```python
from build123d import *

# Parameters (mm, degrees)
BOSS_EXTRUDE1_DEPTH = 1.5875
SKETCH3_R           = 1.5
CUT_EXTRUDE1_DEPTH  = 1.5875
SKETCH4_W           = 8.5
SKETCH4_H           = 40
CUT_EXTRUDE2_DEPTH  = 52.910426175
CUT_EXTRUDE3_DEPTH  = 52.910426175


with BuildPart() as part:
    # Sketch2 → Boss-Extrude1 (new body)
    with BuildSketch(Plane.XY):
        with BuildLine():
            Line((41.075, 26.06487963), (34.753871084, 26.06487963))
            Line((34.753871084, 26.06487963), (34.753871084, 27.4075156))
            ThreePointArc((34.753871084, 27.4075156), (34.460977865, 28.114622381), (33.753871084, 28.4075156))
            Line((33.753871084, 28.4075156), (-33.743187521, 28.4075156))
            ThreePointArc((-33.743187521, 28.4075156), (-34.450294302, 28.114622381), (-34.743187521, 27.4075156))
            Line((-34.743187521, 27.4075156), (-34.743187521, 26.06487963))
            Line((-34.743187521, 26.06487963), (-41.075, 26.06487963))
            Line((-41.075, 26.06487963), (-41.075, 14.733067151))
            Line((-41.075, 14.733067151), (-42.4124996, 14.733067151))
            ThreePointArc((-42.4124996, 14.733067151), (-43.119606381, 14.440173932), (-43.4124996, 13.733067151))
            Line((-43.4124996, 13.733067151), (-43.4124996, -13.743187521))
            ThreePointArc((-43.4124996, -13.743187521), (-43.119606381, -14.450294302), (-42.4124996, -14.743187521))
            Line((-42.4124996, -14.743187521), (-41.075, -14.743187521))
            Line((-41.075, -14.743187521), (-41.075, -26.08512037))
            Line((-41.075, -26.08512037), (-29.75263109, -26.08512037))
            Line((-29.75263109, -26.08512037), (-29.75263109, -27.41690205))
            ThreePointArc((-29.75263109, -27.41690205), (-29.459737872, -28.124008831), (-28.75263109, -28.41690205))
            Line((-28.75263109, -28.41690205), (28.813455755, -28.41690205))
            ThreePointArc((28.813455755, -28.41690205), (29.520562536, -28.124008831), (29.813455755, -27.41690205))
            Line((29.813455755, -27.41690205), (29.813455755, -26.08512037))
            Line((29.813455755, -26.08512037), (41.075, -26.08512037))
            Line((41.075, -26.08512037), (41.075, -19.823575131))
            Line((41.075, -19.823575131), (42.412577294, -19.823575131))
            ThreePointArc((42.412577294, -19.823575131), (43.119684076, -19.530681912), (43.412577294, -18.823575131))
            Line((43.412577294, -18.823575131), (43.412577294, 18.721630511))
            ThreePointArc((43.412577294, 18.721630511), (43.119684076, 19.428737292), (42.412577294, 19.721630511))
            Line((42.412577294, 19.721630511), (41.075, 19.721630511))
            Line((41.075, 19.721630511), (41.075, 26.06487963))
        make_face()
    extrude(amount=BOSS_EXTRUDE1_DEPTH)

    # Sketch3 → Cut-Extrude1 (cut)
    with BuildSketch(Plane(origin=(0, 0, 0), x_dir=(-1, 0, 0), z_dir=(0, 0, -1))):
        with Locations((40.825, 25.825)):
            Circle(SKETCH3_R)
        with Locations((-40.825, 25.825)):
            Circle(SKETCH3_R)
        with Locations((-40.825, -25.825)):
            Circle(SKETCH3_R)
        with Locations((40.825, -25.825)):
            Circle(SKETCH3_R)
    extrude(amount=-CUT_EXTRUDE1_DEPTH, mode=Mode.SUBTRACT)

    # Sketch4 → Cut-Extrude2 (cut, through all)
    with BuildSketch(Plane(origin=(0, 0, 0), x_dir=(-1, 0, 0), z_dir=(0, 0, -1))):
        Polygon((-28.41, -20.51), (-28.41, 20.96), (34.89, 20.96), (34.89, -20.51), (34.89, -22.36), (-28.41, -22.36), align=None)
        with Locations((-34.015313808, 0.1)):
            Rectangle(SKETCH4_W, SKETCH4_H)
    extrude(amount=-CUT_EXTRUDE2_DEPTH, mode=Mode.SUBTRACT)

    # Sketch6 → Cut-Extrude3 (cut, through all)
    with BuildSketch(Plane(origin=(0, 0, 0), x_dir=(-1, 0, 0), z_dir=(0, 0, -1))):
        with BuildLine():
            Line((16.422031316, 26.18), (-4.280813202, 26.18))
            ThreePointArc((-4.280813202, 26.18), (-4.811143288, 25.960330086), (-5.030813202, 25.43))
            Line((-5.030813202, 25.43), (-5.030813202, 20.96))
            Line((-5.030813202, 20.96), (17.172031316, 20.96))
            Line((17.172031316, 20.96), (17.172031316, 25.43))
            ThreePointArc((17.172031316, 25.43), (16.952361402, 25.960330086), (16.422031316, 26.18))
        make_face()
        with BuildLine():
            Line((-2.978741709, -22.36), (9.619202587, -22.36))
            Line((9.619202587, -22.36), (9.619202587, -24.4))
            ThreePointArc((9.619202587, -24.4), (9.472755977, -24.753553391), (9.119202587, -24.9))
            Line((9.119202587, -24.9), (-2.478741709, -24.9))
            ThreePointArc((-2.478741709, -24.9), (-2.832295099, -24.753553391), (-2.978741709, -24.4))
            Line((-2.978741709, -24.4), (-2.978741709, -22.36))
        make_face()
    extrude(amount=-CUT_EXTRUDE3_DEPTH, mode=Mode.SUBTRACT)


solid = part.part
```
For this review, take the finished solid that the model builds, in its own axes (mm). A direction names the side the tool comes from. Give positions to 0.01 mm unless a question says otherwise; leave off trailing zeros. Loops run counter-clockwise (first coordinate to the right, second up) from the corner with the lowest first, then second, coordinate; pieces in that order, holes last. Notation, with made-up numbers: M 57,60.5 L 109,60.5 A26 cw 109,83.5 Z; hole C 83,-30 d11. An arc over 180 degrees is marked long. One line per item, written item: value. Start each with the question number.
Q1. Add section B-B (y = -21.5). Give the boundary of the cut face in (x, z) (1 decimal), and give its area (3 significant figures).
Q2. Add section D-D (z = 1). Count the separate pieces of the cut face and the enclosed holes in it, and give its area (3 significant figures).
Q3. Clearance check with flat-ended pins moving along their axes: pin 1 Ø0.7 at (x, z) = (41.5, 0.5) entering from +Y; pin 2 Ø0.8 at (x, z) = (-33.5, 1) entering from -Y; pin 3 Ø12 at (x, y) = (18, 11) entering from +Z; pin 4 Ø0.7 at (y, z) = (-26.5, 1) entering from -X. State where each tip first meets the part, or that it passes through.
Q4. Add section A-A (y = -2). Give the boundary of the cut face in (x, z).
Q5. Add section C-C (x = -24.5). Give the boundary of the cut face in (y, z).
Q6. For L1, parallel to X at y = 13, z = 0.7; L2, parallel to X at y = 18, z = 0.15 (3 decimals); L3, parallel to Y at x = 32.5, z = 0.6, list the stretches that pass through material, from the lowest coordinate up.
Q7. Machinability: for faces 1 (the face through (35, -26.085, 1)), 2 (the face through (37, 26.065, 1)), 3 (the face through (-17.172, 23, 1)), which of the approach directions +Z, -Z, +X, -X, +Y, -Y give a long, thin tool a straight path to every point of the face, cutting with its end or side? Answer none if there is none.
Q8. Draft analysis for pull direction Y (two halves, no side actions). For faces 4 (the face through (34, -19.9, 1)), 5 (the face through (-41.075, -19, 1)), 6 (the face through (-37, 26.065, 1)), 7 (the face through (38.265, 0, 1)), state which applies: released by +Y, released by -Y, zero draft, split by the parting line, or undercut.
Reply:
1. outline: M -41.1,0 L -34.9,0 L -34.9,1.6 L -41.1,1.6 Z; M 28.4,0 L 41.1,0 L 41.1,1.6 L 28.4,1.6 Z
1. area: 29.9 mm²
2. separate pieces: 1
2. enclosed holes: 2
2. area: 1,510 mm²
3. pin 1: y = 19.72
3. pin 2: y = -26.09
3. pin 3: through
3. pin 4: x = -29.75
4. outline: M -43.41,0 L -34.89,0 L -34.89,1.59 L -43.41,1.59 Z; M 28.41,0 L 29.77,0 L 29.77,1.59 L 28.41,1.59 Z; M 38.27,0 L 43.41,0 L 43.41,1.59 L 38.27,1.59 Z
5. outline: M -28.42,0 L -22.36,0 L -22.36,1.59 L -28.42,1.59 Z; M 20.96,0 L 28.41,0 L 28.41,1.59 L 20.96,1.59 Z
6. L1: -43.41 to -34.89, 28.41 to 29.77, 38.27 to 43.41
6. L2: -41.075 to -34.89, 28.41 to 29.765, 38.265 to 43.413
6. L3: -26.09 to -19.9, 20.1 to 28.41
7. face 1: +Z, -Z, +X, -Y
7. face 2: +Z, -Z, +X, +Y
7. face 3: +Z, -Z
8. face 4: undercut
8. face 5: zero draft
8. face 6: released by +Y
8. face 7: undercut
